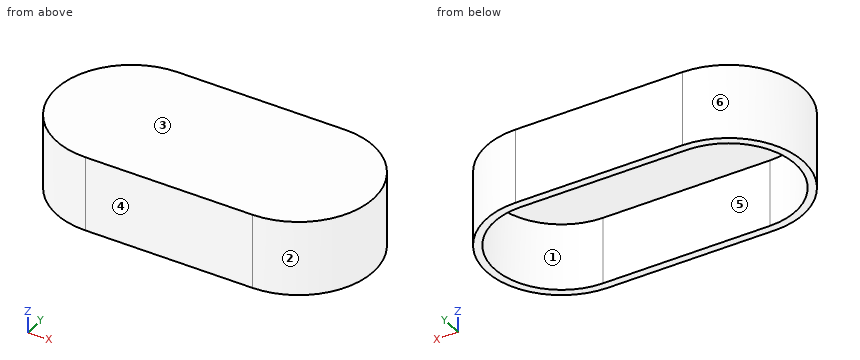
from build123d import *

# Parameters (mm, degrees)
PAD004_DEPTH = 2
PAD_DEPTH    = 15
PAD001_DEPTH = 4


with BuildPart() as topinside:
    # Sketch004 → Pad004 (new body)
    with BuildSketch(Plane.XY.offset(13)):
        with BuildLine():
            ThreePointArc((-21, 17), (-38, 0), (-21, -17))
            Line((-21, -17), (21, -17))
            ThreePointArc((21, -17), (38, 0), (21, 17))
            Line((-21, 17), (21, 17))
        make_face()
    extrude(amount=PAD004_DEPTH)


with BuildPart() as sides:
    # Sketch → Pad (new body)
    with BuildSketch(Plane.XY):
        with BuildLine():
            ThreePointArc((-21, 19), (-40, 0), (-21, -19))
            Line((-21, -19), (21, -19))
            ThreePointArc((21, -19), (40, 0), (21, 19))
            Line((-21, 19), (21, 19))
        make_face()
        with BuildLine():
            ThreePointArc((-21, 17), (-38, 0), (-21, -17))
            Line((-21, -17), (21, -17))
            ThreePointArc((21, -17), (38, 0), (21, 17))
            Line((-21, 17), (21, 17))
        make_face(mode=Mode.SUBTRACT)
    extrude(amount=PAD_DEPTH)


with BuildPart() as sides_1:
    # Body placement: moved
    add(sides.part.moved(Location((0, 0, -2))))


with BuildPart() as top:
    # Sketch001 → Pad001 (new body)
    with BuildSketch(Plane.XY.offset(13)):
        with BuildLine():
            ThreePointArc((-21, 19), (-40, 0), (-21, -19))
            Line((-21, -19), (21, -19))
            ThreePointArc((21, -19), (40, 0), (21, 19))
            Line((-21, 19), (21, 19))
        make_face()
    extrude(amount=PAD001_DEPTH)

    # Boolean: cut TopInside
    add(topinside.part, mode=Mode.SUBTRACT)

    # Boolean002: union Sides
    add(sides_1.part)


solid = top.part
Work out the finished part from the listing and answer in its coordinate system (mm). Face numbers are marked on the shaded views. A direction names the side the tool comes from. Give positions to 0.01 mm unless a question says otherwise; leave off trailing zeros. Loops run counter-clockwise (first coordinate to the right, second up) from the corner with the lowest first, then second, coordinate; pieces in that order, holes last. Notation, with made-up numbers: (38.25, 77.5) -> (45.25, 77.5) arc R26 ccw to (45.25, 108.5) -> close; hole circle Ø7 at (-39.5, -1.75). An arc over 180 degrees is marked (long way). Use a Markdown table: item, result. Add a question column.
1. Determine the mould class of the marked faces 3, 4, 5 and 6 for opening direction Y: released by +Y, released by -Y, zero draft, split by the parting line, or undercut.
2. Find the intervals of material crossed by probe 1 along Y at (x, z) = (-13.5, 14); probe 2 along X at (y, z) = (-0.5, 0.25); probe 3 along Z at (x, y) = (-24.5, 3), in increasing order.
3. Section B-B on z = 6.5 is taken. Determine the outline of the cut face in (x, y), and give its area (3 significant figures).
4. Flat-ended cylindrical pins translate along their axes: pin 1 Ø2 at (x, z) = (-29, 9) entering from +Y; pin 2 Ø2 at (x, z) = (23, 14.5) entering from +Y; pin 3 Ø4 at (y, z) = (-1.5, 6) entering from +X. Find the tip coordinate at first contact, or state that the pin passes through.
5. For the marked faces 1 and 2, determine the directions among +Z, -Z, +X, -X, +Y, -Y from which every point of the face is accessible in a straight line to the end or side of a thin tool.
6. Section A-A on x = 0 is taken. Determine the outline of the cut face in (y, z).
7. Section C-C on y = 0 is taken. Determine the outline of the cut face in (x, z).
Results below:
| question | item | result |
|---|---|---|
| 1 | face 3 | zero draft |
| 1 | face 4 | released by -Y |
| 1 | face 5 | undercut |
| 1 | face 6 | split by the parting line |
| 2 | probe 1 | y = -19 to -17, 17 to 19 |
| 2 | probe 2 | x = -39.99 to -37.99, 37.99 to 39.99 |
| 2 | probe 3 | z = 15 to 17 |
| 3 | outline | (-21, -19) -> (21, -19) arc R19 ccw to (21, 19) -> (-21, 19) arc R19 ccw to start; hole (-21, -17) -> (21, -17) arc R17 ccw to (21, 17) -> (-21, 17) arc R17 ccw to start |
| 3 | area | 394 mm^2 |
| 4 | pin 1 | stops at y = 17.66 |
| 4 | pin 2 | stops at y = 18.97 |
| 4 | pin 3 | stops at x = 40 |
| 5 | face 1 | -Z |
| 5 | face 2 | +Z, -Z, +X |
| 6 | outline | (-19, -2) -> (-17, -2) -> (-17, 15) -> (17, 15) -> (17, -2) -> (19, -2) -> (19, 17) -> (-19, 17) -> close |
| 7 | outline | (-40, -2) -> (-38, -2) -> (-38, 15) -> (38, 15) -> (38, -2) -> (40, -2) -> (40, 17) -> (-40, 17) -> close |
